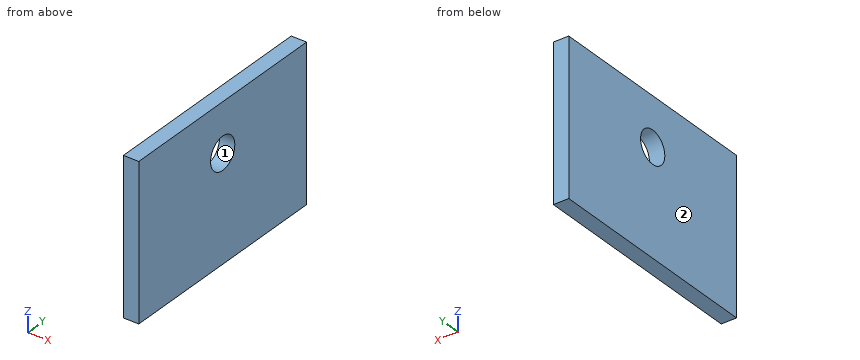
Autodesk Inventor part; units mm, degrees
ref_plane "YZ Plane" through (0, 0, 0) normal (1, 0, 0) x (0, 1, 0)
ref_plane "XZ Plane" through (0, 0, 0) normal (0, 1, 0) x (-1, 0, 0)
ref_plane "XY Plane" through (0, 0, 0) normal (0, 0, 1) x (1, 0, 0)
sketch "Sketch1" plane through (0, 0, 0) normal (1, 0, 0) x (0, 1, 0)
  line L0 (0, 0) -> (88, 0)
  line L1 (88, 0) -> (88, 60)
  line L2 (88, 60) -> (0, 60)
  line L3 (0, 60) -> (0, 0)
  dimension "d0" = 88
  dimension "d1" = 60
extrude "Extrusion1" add sketch "Sketch1" along normal blind 6
sketch "Sketch2" plane through (0, 0, 0) normal (-1, 0, 0) x (0, 0, 1)
  line L0 (60, 0) -> (0, 0)
  line L1 (0, 0) -> (0, 88)
  circle A0 centre (41, 44) radius 6.35
  dimension "d4" = 44
  dimension "d5" = 41
  dimension "d6" = 12.7
extrude "Extrusion2" cut sketch "Sketch2" against normal blind 6
properties part number "motor_base"
Geometry check sheet. Reference: the model listing, model coordinates, mm. Face numbers are marked on the shaded views. Round coordinates to 2 decimals unless told otherwise and drop trailing zeros. Loops run counter-clockwise (first coordinate to the right, second up) from the corner with the lowest first, then second, coordinate; pieces in that order, holes last. Notation, with made-up numbers: (43, 24) -> (50, 24) arc R23 ccw to (50, 40) -> close; hole circle Ø7 at (-24, -2.5). An arc over 180 degrees is marked (long way). Answer as a JSON object with one key per item and string values. Group by question number.
Item 1: Cross-section at A-A, the plane y = 44. Record the cut outline in (x, z).
Item 2: Depth check by flat-ended pin: pin 1 Ø1.5 at (y, z) = (46, 36.5) entering from -X. Enter the tip coordinate at first touch or a pass-through.
Item 3: Release check for a two-part mould opening along Z. For the marked faces 1 and 2 record: pulls with the +Z half, pulls with the -Z half, needs draft (parallel to the pull), parting line crosses it, or undercut.
Item 4: Cross-section at B-B, the plane z = 41. Record the cut outline in (x, y), plus the area to 3 significant figures.
Item 5: Thickness scan on line 1 along Y through (x, z) = (4, 41); line 2 along Y through (x, z) = (3.65, 37); line 3 along Z through (x, y) = (2.7, 48.5). Record the ranges inside material, lowest first.
Item 6: Cross-section at C-C, the plane x = 2.15. Record the cut outline in (y, z), plus the area to 3 significant figures.
Determined:
{
 "1": {"outline": "(0, 0) -> (6, 0) -> (6, 34.65) -> (0, 34.65) -> close; (0, 47.35) -> (6, 47.35) -> (6, 60) -> (0, 60) -> close"},
 "2": {"pin 1": "passes through"},
 "3": {"face 1": "undercut", "face 2": "needs draft"},
 "4": {"outline": "(0, 0) -> (6, 0) -> (6, 37.65) -> (0, 37.65) -> close; (0, 50.35) -> (6, 50.35) -> (6, 88) -> (0, 88) -> close", "area": "452 mm²"},
 "5": {"line 1": "y = 0 to 37.65, 50.35 to 88", "line 2": "y = 0 to 39.07, 48.93 to 88", "line 3": "z = 0 to 36.52, 45.48 to 60"},
 "6": {"outline": "(0, 0) -> (88, 0) -> (88, 60) -> (0, 60) -> close; hole circle Ø12.7 at (44, 41)", "area": "5,150 mm²"}
}
